```python
from build123d import *

# Parameters (mm, degrees)
F0_W      = 38.3663107641
F0_H      = 42.2096475959
F1_DEPTH  = 0.6858
F3_W      = 400
F3_H      = 305
F4_DEPTH  = 5
F5_W      = 5
F5_H      = 305
F6_DEPTH  = 20
F7_W      = 5
F7_H      = 305
F8_DEPTH  = 20
F9_W      = 400
F9_H      = 25
F10_DEPTH = 5
F11_W     = 5
F11_H     = 305
F12_DEPTH = 20
F13_W     = 400
F13_H     = 25
F14_DEPTH = 5
F15_R     = 5
F16_DEPTH = 10
F17_R     = 7.5
F17_R_2   = 5
F18_DEPTH = 10


with BuildPart() as f1:
    # F0 (on Top) → F1 (new body)
    with BuildSketch(Plane.XY):
        with Locations((-14.0401979443, 21.1048237979)):
            Rectangle(F0_W, F0_H)
    extrude(amount=F1_DEPTH)


with BuildPart() as f4:
    # F3 (on Top) → F4 (new body)
    with BuildSketch(Plane.XY):
        Rectangle(F3_W, F3_H)
    extrude(amount=F4_DEPTH)

    # F5 (on face) → F6 (join)
    with BuildSketch(Plane.XY.offset(5)):
        with Locations((-197.5, 0)):
            Rectangle(F5_W, F5_H)
    extrude(amount=F6_DEPTH)

    # F7 (on face) → F8 (join)
    with BuildSketch(Plane.XY.offset(5)):
        with Locations((197.5, 0)):
            Rectangle(F7_W, F7_H)
    extrude(amount=F8_DEPTH)

    # F9 (on face) → F10 (join)
    with BuildSketch(Plane(origin=(0, 152.5, 0), x_dir=(-1, 0, 0), z_dir=(0, 1, 0))):
        with Locations((0, 12.5)):
            Rectangle(F9_W, F9_H)
    extrude(amount=F10_DEPTH)

    # F11 (on face) → F12 (join)
    with BuildSketch(Plane.XY.offset(5)):
        Rectangle(F11_W, F11_H)
    extrude(amount=F12_DEPTH)

    # F13 (on face) → F14 (join)
    with BuildSketch(Plane.XZ.offset(152.5)):
        with Locations((0, 12.5)):
            Rectangle(F13_W, F13_H)
    extrude(amount=F14_DEPTH)

    # F15 (on face) → F16 (join)
    with BuildSketch(Plane.XZ.offset(157.5)):
        with Locations((0, 12.090690434)):
            Circle(F15_R)
    extrude(amount=F16_DEPTH)

    # F17 (on face) → F18 (join)
    with BuildSketch(Plane.XZ.offset(167.5)):
        with Locations((0, 12.090690434)):
            Circle(F17_R)
        with Locations((0, 12.090690434)):
            Circle(F17_R_2, mode=Mode.SUBTRACT)
        with Locations((0, 12.090690434)):
            Circle(F17_R_2)
    extrude(amount=F18_DEPTH)


solid = f4.part
```
Can you work these out from the model? Positions are in its coordinate system, mm. A direction names the side the tool comes from. Coordinates: 2 decimals unless noted, no trailing zeros. Order: outer loops, then holes, each group sorted by start corner. A loop starts at its lowest first (then second) coordinate and runs counter-clockwise, first axis right, second up. Notation, with made-up numbers: (34, -24) -> (61, -24) arc R32 ccw to (61, 13) -> close; hole circle Ø5 at (64.5, 16.5). An arc over 180 degrees is marked (long way). Write each question's results on one line, items separated by ' | '.
Item 1: I want a section at A-A, the plane x = 40. Write out the boundary of the cut face in (y, z), then the cut area to 4 significant figures.
Results are:
outline: (-157.5, 0) -> (157.5, 0) -> (157.5, 25) -> (152.5, 25) -> (152.5, 5) -> (-152.5, 5) -> (-152.5, 25) -> (-157.5, 25) -> close | area: 1,775 mm²
Item 2: I'm going to push flat-ended pins straight in: pin 1 Ø1.5 at (x, y) = (-87, -76) entering from +Z; pin 2 Ø4 at (x, z) = (159.5, 17.5) entering from -Y. Where does each tip first touch, or does it pass through?
Results are:
pin 1: z = 5 | pin 2: y = -157.5
Item 3: Which directions (+Z, -Z, +X, -X, +Y, -Y) give clear straight access to the entire face, cutting with the end or side of a thin tool? Please do faces 1 (the face through (-100, -152.5, 15)), 2 (the face through (-1.63, -172.43, 4.77)), 3 (the face through (4.9, -167.5, 10.5)), 4 (the face through (-1, 1, 25)).
Results are:
face 1: +Z | face 2: -Y | face 3: none | face 4: +Z, +X, -X, +Y, -Y
Item 4: If we mould it in two halves opening along Y, with no side actions, what happens to faces 5 (the face through (3, 157.5, 13)), 6 (the face through (97, 2, 5)), 7 (the face through (-1.08, -162.43, 7.21)), 8 (the face through (0, -177.5, 12))? For each: +Y half, -Y half, draft (parallel to the pull), parting line (faces both ways), or undercut.
Results are:
face 5: +Y half | face 6: undercut | face 7: undercut | face 8: -Y half
Item 5: If I drill on line 1 along X through (y, z) = (138, 19.25); line 2 along Y through (x, z) = (7, 16.25); line 3 along Z through (x, y) = (-139, -89), over which ranges is the centre line in solid material (lowest first)?
Results are:
line 1: -200 to -195, -2.5 to 2.5, 195 to 200 | line 2: -157.5 to -152.5, 152.5 to 157.5 | line 3: 0 to 5
Item 6: I want a section at B-B, the plane y = -47. Write out the boundary of the cut face in (x, z).
Results are:
outline: (-200, 0) -> (200, 0) -> (200, 25) -> (195, 25) -> (195, 5) -> (2.5, 5) -> (2.5, 25) -> (-2.5, 25) -> (-2.5, 5) -> (-195, 5) -> (-195, 25) -> (-200, 25) -> close
